Part model, mm, in its own coordinate system. Round coordinates to 2 decimals unless told otherwise and drop trailing zeros. Write each loop counter-clockwise with the first axis right and the second up, starting at its lowest first coordinate (ties: lowest second). Pieces come first, ordered by that corner, then holes. Notation, with made-up numbers: (-9.5, 41.5) -> (19.5, 41.5) arc R27 ccw to (19.5, 69.5) -> close; hole circle Ø8 at (-13, 1). An arc over 180 degrees is marked (long way). Use CSV: the item, a comma, the result in double quotes. Start each with the question number.
(1) Drop flat-ended pins along their axis: pin 1 (4 mm diameter, centred on y = -4, z = 165.5, fed in from +X); pin 2 (5 mm diameter, centred on y = 5.5, z = 97.5, fed in from +X); pin 3 (10 mm diameter, centred on y = 8.5, z = 167, fed in from +X); pin 4 (8 mm diameter, centred on x = -1, y = -6.5, fed in from +Z). Give the stop position or say it passes through.
(2) Saw through at B-B (x = 3.5). Give the cut face in (y, z), plus the area to 3 significant figures.
(3) Saw through at C-C (z = 168.5). Give the cut face in (x, y).
(4) Saw through at A-A (y = 0). Give the cut face in (x, z), plus the area to 3 significant figures.
(5) Probe line 1 (Y direction, x = 0, z = 67); line 2 (Y direction, x = 6.5, z = 213.5); line 3 (X direction, y = 0.5, z = 90). List the from-to ranges inside material, lowest first. Write a range as [from, to].
```python
from build123d import *

# Parameters (mm, degrees)
SKETCH_1_R          = 12.5
EXTRUDE_2_DEPTH     = 235.43
SKETCH_2_R          = 9
CUT_EXTRUDE_1_DEPTH = 235.43
EXTRUDE_START       = 15.57
SKETCH_3_R          = 12.5
EXTRUDE_3_DEPTH     = 15.57
SKETCH_4_R          = 9
CUT_EXTRUDE_2_DEPTH = 20
EXTRUDE_START_2     = 9.93
SKETCH_5_R          = 12.5
EXTRUDE_4_DEPTH     = 9.93
SKETCH_6_R          = 9
CUT_EXTRUDE_3_DEPTH = 10
SKETCH_7_R          = 26.85848727
CUT_EXTRUDE_4_DEPTH = 14.93
SKETCH_8_R          = 12.5
EXTRUDE_5_DEPTH     = 9.93
SKETCH_9_R          = 9
CUT_EXTRUDE_5_DEPTH = 10
SKETCH_10_R         = 37.193394561
CUT_EXTRUDE_6_DEPTH = 0.22
SKETCH_11_R         = 43.187188263
CUT_EXTRUDE_7_DEPTH = 0.71
SKETCH_12_R         = 11
CUT_EXTRUDE_8_DEPTH = 338


with BuildPart() as part:
    # 草图1 → 凸台-拉伸2 (new body)
    with BuildSketch(Plane.XY):
        Circle(SKETCH_1_R)
    extrude(amount=EXTRUDE_2_DEPTH)

    # 草图2 → 切除-拉伸1 (cut)
    with BuildSketch(Plane(origin=(0, 0, 0), x_dir=(-1, 0, 0), z_dir=(0, 0, -1))):
        Circle(SKETCH_2_R)
    extrude(amount=-CUT_EXTRUDE_1_DEPTH, mode=Mode.SUBTRACT)

    # 草图3 → 凸台-拉伸3 (add)
    with BuildSketch(Plane(origin=(0, 0, 0), x_dir=(-1, 0, 0), z_dir=(0, 0, -1)).offset(EXTRUDE_START)):
        Circle(SKETCH_3_R)
    extrude(amount=-EXTRUDE_3_DEPTH)

    # 草图4 → 切除-拉伸2 (cut)
    with BuildSketch(Plane(origin=(0, 0, -15.57), x_dir=(-1, 0, 0), z_dir=(0, 0, -1))):
        Circle(SKETCH_4_R)
    extrude(amount=-CUT_EXTRUDE_2_DEPTH, mode=Mode.SUBTRACT)

    # 草图5 → 凸台-拉伸4 (add)
    with BuildSketch(Plane(origin=(0, 0, -15.57), x_dir=(-1, 0, 0), z_dir=(0, 0, -1)).offset(EXTRUDE_START_2)):
        Circle(SKETCH_5_R)
    extrude(amount=-EXTRUDE_4_DEPTH)

    # 草图6 → 切除-拉伸3 (cut)
    with BuildSketch(Plane(origin=(0, 0, -25.5), x_dir=(-1, 0, 0), z_dir=(0, 0, -1))):
        Circle(SKETCH_6_R)
    extrude(amount=-CUT_EXTRUDE_3_DEPTH, mode=Mode.SUBTRACT)

    # 草图7 → 切除-拉伸4 (cut)
    with BuildSketch(Plane(origin=(0, 0, -25.5), x_dir=(-1, 0, 0), z_dir=(0, 0, -1))):
        Circle(SKETCH_7_R)
    extrude(amount=-CUT_EXTRUDE_4_DEPTH, mode=Mode.SUBTRACT)

    # 草图8 → 凸台-拉伸5 (add)
    with BuildSketch(Plane(origin=(0, 0, -10.57), x_dir=(-1, 0, 0), z_dir=(0, 0, -1)).offset(EXTRUDE_START_2)):
        Circle(SKETCH_8_R)
    extrude(amount=-EXTRUDE_5_DEPTH)

    # 草图9 → 切除-拉伸5 (cut)
    with BuildSketch(Plane(origin=(0, 0, -20.5), x_dir=(-1, 0, 0), z_dir=(0, 0, -1))):
        Circle(SKETCH_9_R)
    extrude(amount=-CUT_EXTRUDE_5_DEPTH, mode=Mode.SUBTRACT)

    # 草图10 → 切除-拉伸6 (cut)
    with BuildSketch(Plane(origin=(0, 0, -20.5), x_dir=(-1, 0, 0), z_dir=(0, 0, -1))):
        with Locations((7.201744855, 7.507888779)):
            Circle(SKETCH_10_R)
    extrude(amount=-CUT_EXTRUDE_6_DEPTH, mode=Mode.SUBTRACT)

    # 草图11 → 切除-拉伸7 (cut)
    with BuildSketch(Plane(origin=(0, 0, -20.28), x_dir=(-1, 0, 0), z_dir=(0, 0, -1))):
        with Locations((-1.225460352, 2.329416421)):
            Circle(SKETCH_11_R)
    extrude(amount=-CUT_EXTRUDE_7_DEPTH, mode=Mode.SUBTRACT)

    # 草图12 → 切除-拉伸8 (cut)
    with BuildSketch(Plane(origin=(0, 0, -19.57), x_dir=(-1, 0, 0), z_dir=(0, 0, -1))):
        Circle(SKETCH_12_R)
    extrude(amount=-CUT_EXTRUDE_8_DEPTH, mode=Mode.SUBTRACT)


solid = part.part
```
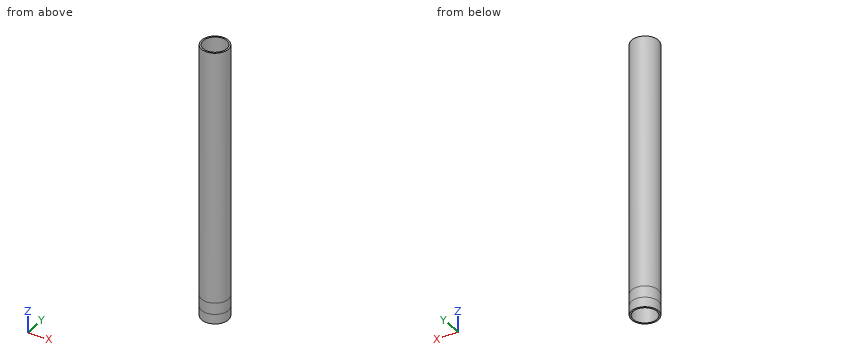
Answers:
1,pin 1,"stops at x = 12.34"
1,pin 2,"stops at x = 12.13"
1,pin 3,"stops at x = 12"
1,pin 4,"passes through"
2,outline,"(-12, -19.57) -> (-10.43, -19.57) -> (-10.43, 235.43) -> (-12, 235.43) -> close; (10.43, -19.57) -> (12, -19.57) -> (12, 235.43) -> (10.43, 235.43) -> close"
2,area,"802 mm²"
3,outline,"circle Ø25 at (0, 0); hole circle Ø22 at (0, 0)"
4,outline,"(-12.5, -19.57) -> (-11, -19.57) -> (-11, 235.43) -> (-12.5, 235.43) -> close; (11, -19.57) -> (12.5, -19.57) -> (12.5, 235.43) -> (11, 235.43) -> close"
4,area,"765 mm²"
5,line 1,"y = [-12.5, -11], [11, 12.5]"
5,line 2,"y = [-10.68, -8.87], [8.87, 10.68]"
5,line 3,"x = [-12.49, -10.99], [10.99, 12.49]"
